Could you check a few things on this drawing? It's one solid part, dimensions in mm from its lowest x, y, z. A direction names the side the tool comes from. Give positions to 0.01 mm unless a question says otherwise; leave off trailing zeros. Write each loop counter-clockwise with the first axis right and the second up, starting at its lowest first coordinate (ties: lowest second). Pieces come first, ordered by that corner, then holes. Notation, with made-up numbers: M 30,7 L 61,7 A28 cw 61,25 Z; hole C -38.75,62.5 d10. An arc over 180 degrees is marked long. Answer as CSV lines item,"result". Start each with the question number.
Q1. For pin 1 (2 mm diameter, centred on x = 11, y = 5, fed in from -Z); pin 2 (1 mm diameter, centred on y = 1, z = 21, fed in from -X); pin 3 (6 mm diameter, centred on x = 15, z = 15, fed in from +Y), each with a flat end and sliding along its axis, tell me the tip position at first contact or that it passes through.
Q2. Suppose I cut it at C-C (y = 4.25). Write out the boundary of the cut face in (x, z).
Q3. Suppose I cut it at D-D (z = 6.75). Write out the boundary of the cut face in (x, y).
Q4. Suppose I cut it at B-B (x = 15). Write out the boundary of the cut face in (y, z), then the cut area to 3 significant figures.
Q5. If I drill on line 1 along Z through (x, y) = (15, 6.75); line 2 along X through (y, z) = (4.25, 16.5); line 3 along Y through (x, z) = (15.25, 25.75), over which ranges is the centre line in solid material (lowest first)?
Q6. On a 3-axis mill with a long thin cutter (end or side, diameter ignored), from which of +Z, -Z, +X, -X, +Y, -Y can I reach the whole of each face in a straight line? I mean the marked faces 1 and 2. Say none if no direction works.
Q7. Suppose I cut it at A-A (z = 15). Write out the boundary of the cut face in (x, y).
Q8. Thinking about a two-plate mould opening in X: for the marked faces 3, 4 and 5, which applies, +X half, -X half, draft (parallel to the pull), parting line (faces both ways), or undercut?
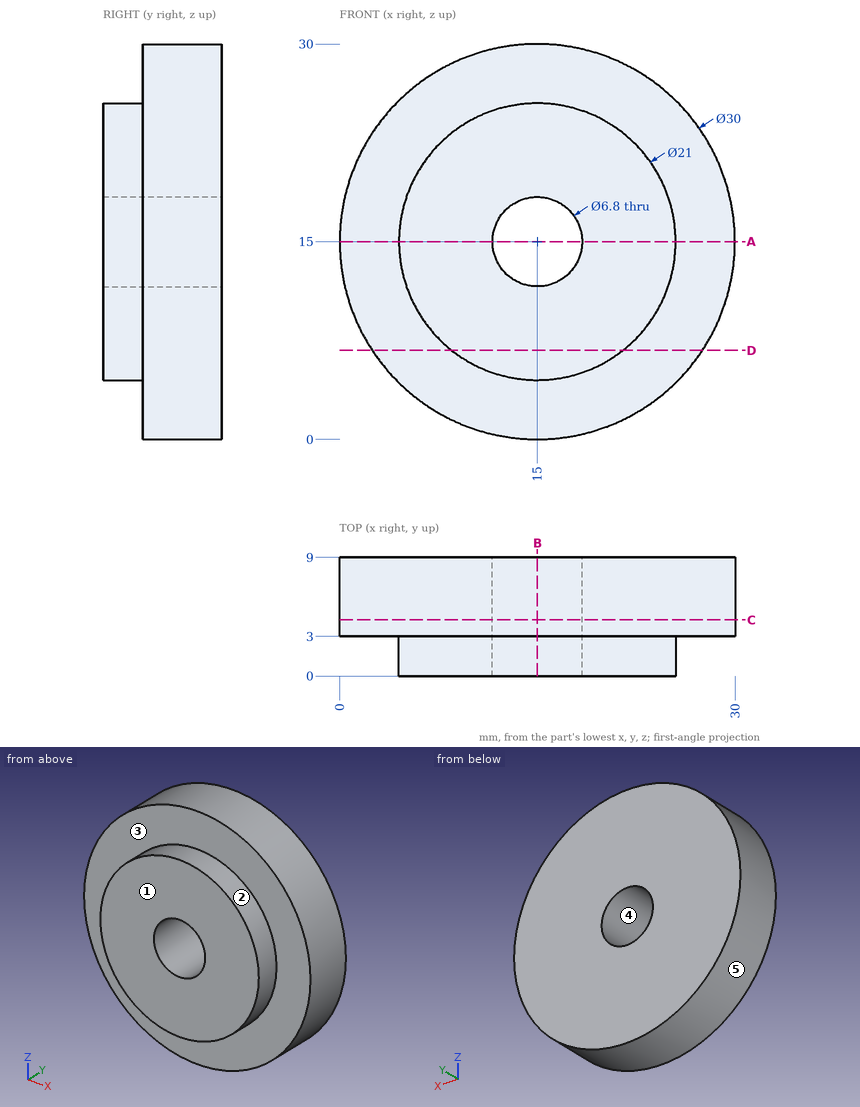
Resolved:
1,pin 1,"z = 0.3"
1,pin 2,"x = 6.06"
1,pin 3,"through"
2,outline,"C 15,15 d30; hole C 15,15 d6.8"
3,outline,"M 2.47,3 L 8.5,3 L 8.5,0 L 21.5,0 L 21.5,3 L 27.53,3 L 27.53,9 L 2.47,9 Z"
4,outline,"M 0,4.5 L 3,4.5 L 3,0 L 9,0 L 9,11.6 L 0,11.6 Z; M 0,18.4 L 9,18.4 L 9,30 L 3,30 L 3,25.5 L 0,25.5 Z"
4,area,"182 mm^2"
5,line 1,"0 to 11.6, 18.4 to 30"
5,line 2,"0.08 to 11.95, 18.05 to 29.92"
5,line 3,"3 to 9"
6,face 1,"+Z, -Z, +X, -X, -Y"
6,face 2,"-Y"
7,outline,"M 0,3 L 4.5,3 L 4.5,0 L 11.6,0 L 11.6,9 L 0,9 Z; M 18.4,0 L 25.5,0 L 25.5,3 L 30,3 L 30,9 L 18.4,9 Z"
8,face 3,"draft"
8,face 4,"undercut"
8,face 5,"parting line"
